Source: CAD feature listing. Evaluate the final solid. Frame: model axes, mm. Face numbers are marked on the shaded views. A direction names the side the tool comes from. Give positions to 0.01 mm unless a question says otherwise; leave off trailing zeros. Write each loop counter-clockwise with the first axis right and the second up, starting at its lowest first coordinate (ties: lowest second). Pieces come first, ordered by that corner, then holes. Notation, with made-up numbers: (-35, -6.75) -> (-14, -6.75) arc R16 cw to (-14, -2.75) -> close; hole circle Ø9 at (83, 49). An arc over 180 degrees is marked (long way). Use one line per item in the form item = value. Start each with the question number.
(1) Cut plane D-D, the plane y = 7.5. Output: boundary loops of the cut face in (x, z), and give its area (4 significant figures).
(2) Set-up query: the marked faces 4, 5 and 6. Return all of +Z, -Z, +X, -X, +Y, -Y with unobstructed straight access to the full face (end or side cutting, diameter ignored); none if empty.
(3) Cut plane B-B, the plane z = -4.25. Output: boundary loops of the cut face in (x, y).
(4) Cut plane A-A, the plane y = 0. Output: boundary loops of the cut face in (x, z), and give its area (3 significant figures).
(5) Cut plane C-C, the plane x = -4.5. Output: boundary loops of the cut face in (y, z), and give its area (3 significant figures).
(6) First-contact query: P1, Ø8, axis at x = -1.5, y = -5.5, coming from the -Z side; P2, Ø4, axis at x = -7.5, y = -6.5, coming from the -Z side; P3, Ø10, axis at x = -6.5, y = 7, coming from the -Z side; P4, Ø10, axis at x = 1, z = -8.5, coming from the -Y side. Flat tips, straight axial feed; report the tip coordinate or a pass-through.
(7) Draft query along Y for the marked faces 1, 2 and 3. Return one class per face: pulls with the +Y half, pulls with the -Y half, needs draft (parallel to the pull), parting line crosses it, or undercut.
(8) Material intervals for line 1 along Y through (x, z) = (0, 0.5); line 2 along X through (y, z) = (-3, -19.5); line 3 along X through (y, z) = (-7.5, 0.95), sorted ascending. Write a range as from..to.
from build123d import *

# Parameters (mm, degrees)
SKETCH1_W               = 16
SKETCH1_H               = 18
SKETCH1_W_2             = 12
SKETCH1_H_2             = 14
EXTRUDE_THIN1_DEPTH     = 2
BOSS_EXTRUDE3_DEPTH     = 2.2
CUT_EXTRUDE4_REACH      = 34.067
SKETCH10_W              = 0.2
SKETCH10_H              = 27.531461486
SKETCH5_R               = 3
CUT_EXTRUDE1_DEPTH      = 2
CUT_EXTRUDE1_DRAFT      = -35
MIRROR3_COPY_1_SKETCH_R = 3
MIRROR3_COPY_1_DEPTH    = 2
MIRROR3_COPY_1_DRAFT    = -35
SKETCH14_W              = 12
SKETCH14_H              = 4
BOSS_EXTRUDE5_DEPTH     = 14
CUT_EXTRUDE6_REACH      = 28.292
SKETCH15_R              = 6
CUT_EXTRUDE8_REACH      = 28.292
SKETCH19_R              = 0.5


with BuildPart() as part:
    # Sketch1 → Extrude-Thin1 (new, symmetric)
    with BuildSketch(Plane.XY):
        Rectangle(SKETCH1_W, SKETCH1_H)
        Rectangle(SKETCH1_W_2, SKETCH1_H_2, mode=Mode.SUBTRACT)
    extrude_thin1 = extrude(amount=EXTRUDE_THIN1_DEPTH, both=True)

    # Sketch4 → Boss-Extrude3 (add)
    with BuildSketch(Plane(origin=(8, 0, 0), x_dir=(0, 0, -1), z_dir=(1, 0, 0))):
        with BuildLine():
            Line((-2, 9), (15.5, 9))
            ThreePointArc((15.5, 9), (24.5, 0), (15.5, -9))
            Line((15.5, -9), (-2, -9))
            Line((-2, -9), (-2, 9))
        make_face()
    boss_extrude3 = extrude(amount=BOSS_EXTRUDE3_DEPTH)

    # Sketch10 → Cut-Extrude4 (cut, up to next)
    with BuildSketch(Plane(origin=(0, 9, 0), x_dir=(1, 0, 0), z_dir=(0, 1, 0)), mode=Mode.PRIVATE) as cut_extrude4_sk1:
        with Locations((8.1, 15.765730743)):
            Rectangle(SKETCH10_W, SKETCH10_H)
    cut_extrude4_tool1 = extrude(cut_extrude4_sk1.sketch, amount=-CUT_EXTRUDE4_REACH, mode=Mode.PRIVATE) & part.part
    cut_extrude4 = cut_extrude4_tool1.solids().sort_by_distance((8.1, 9, -15.765731))[0]
    add(cut_extrude4, mode=Mode.SUBTRACT)


with BuildPart() as cut_extrude1_tool:
    # Sketch5 → Cut-Extrude1 (with draft: the straight prism first)
    with BuildSketch(Plane.ZY.offset(-8.2)):
        with Locations((-15.5, 0)):
            Circle(SKETCH5_R)
    extrude(amount=-CUT_EXTRUDE1_DEPTH)
    # Cut-Extrude1: the draft: its side faces are tilted about the plane it starts from
    cut_extrude1_sides = [cut_extrude1_tool.faces().sort_by_distance(p)[0] for p in [
        (9.2, 0, -18.5),
    ]]
    draft(cut_extrude1_sides, Plane.ZY.offset(-8.2), CUT_EXTRUDE1_DRAFT)


with BuildPart() as part_1:
    add(part.part)

    # Cut-Extrude1: cut by cut_extrude1_tool
    add(cut_extrude1_tool.part, mode=Mode.SUBTRACT)

    # Mirror3: Extrude-Thin1, Boss-Extrude3, Cut-Extrude4 across plane
    add(extrude_thin1.mirror(Plane(origin=(0, 0, 0), x_dir=(0, 0, 1), z_dir=(1, 0, 0))))
    add(boss_extrude3.mirror(Plane(origin=(0, 0, 0), x_dir=(0, 0, 1), z_dir=(1, 0, 0))))
    add(cut_extrude4.mirror(Plane(origin=(0, 0, 0), x_dir=(0, 0, 1), z_dir=(1, 0, 0))), mode=Mode.SUBTRACT)


with BuildPart() as mirror3_copy_1_tool:
    # Mirror3 copy 1 sketch → Mirror3 copy 1 (with draft: the straight prism first)
    with BuildSketch(Plane(origin=(-8.2, 0, 0), x_dir=(0, 0, 1), z_dir=(1, 0, 0))):
        with Locations((-15.5, 0)):
            Circle(MIRROR3_COPY_1_SKETCH_R)
    extrude(amount=-MIRROR3_COPY_1_DEPTH)
    # Mirror3 copy 1: the draft: its side faces are tilted about the plane it starts from
    mirror3_copy_1_sides = [mirror3_copy_1_tool.faces().sort_by_distance(p)[0] for p in [
        (-9.2, 0, -18.5),
    ]]
    draft(mirror3_copy_1_sides, Plane(origin=(-8.2, 0, 0), x_dir=(0, 0, 1), z_dir=(1, 0, 0)), MIRROR3_COPY_1_DRAFT)


with BuildPart() as part_2:
    add(part_1.part)

    # Mirror3 copy 1: cut by mirror3_copy_1_tool
    add(mirror3_copy_1_tool.part, mode=Mode.SUBTRACT)

    # Sketch14 → Boss-Extrude5 (add)
    with BuildSketch(Plane(origin=(0, -7, 0), x_dir=(1, 0, 0), z_dir=(0, 1, 0))):
        Rectangle(SKETCH14_W, SKETCH14_H)
    extrude(amount=BOSS_EXTRUDE5_DEPTH)

    # Sketch15 → Cut-Extrude6 (cut, up to next)
    with BuildSketch(Plane(origin=(0, 0, -2), x_dir=(-1, 0, 0), z_dir=(0, 0, -1)), mode=Mode.PRIVATE) as cut_extrude6_sk1:
        Circle(SKETCH15_R)
    cut_extrude6_tool1 = extrude(cut_extrude6_sk1.sketch, amount=-CUT_EXTRUDE6_REACH, mode=Mode.PRIVATE) & part_2.part
    add(cut_extrude6_tool1.solids().sort_by_distance((0, 0, -2))[0], mode=Mode.SUBTRACT)

    # Sketch19 → Cut-Extrude8 (cut, up to next)
    with BuildSketch(Plane(origin=(0, 0, -2), x_dir=(-1, 0, 0), z_dir=(0, 0, -1)), mode=Mode.PRIVATE) as cut_extrude8_sk1:
        with Locations((0, 7.5)):
            Circle(SKETCH19_R)
    cut_extrude8_tool1 = extrude(cut_extrude8_sk1.sketch, amount=-CUT_EXTRUDE8_REACH, mode=Mode.PRIVATE) & part_2.part
    cut_extrude8 = cut_extrude8_tool1.solids().sort_by_distance((0, 7.5, -2))[0]
    add(cut_extrude8, mode=Mode.SUBTRACT)

    # Mirror8: Cut-Extrude8 across plane
    add(cut_extrude8.mirror(Plane.ZX), mode=Mode.SUBTRACT)

    # Mirror8 at the second plane: Cut-Extrude8 across plane
    add(cut_extrude8.mirror(Plane(origin=(0, 0, 0), x_dir=(0, 0, 1), z_dir=(1, 0, 0))), mode=Mode.SUBTRACT)


solid = part_2.part
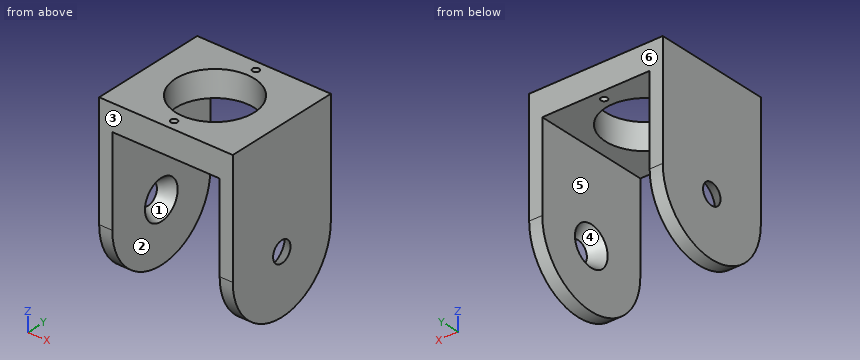
Geometry says:
q1.outline = (-10.2, -20.47) -> (-8.2, -20.47) -> (-8.2, -2) -> (-0.5, -2) -> (-0.5, 2) -> (-10.2, 2) -> close; (0.5, -2) -> (8.2, -2) -> (8.2, -20.47) -> (10.2, -20.47) -> (10.2, 2) -> (0.5, 2) -> close
q1.area = 151.5 mm^2
q2.face_4 = none
q2.face_5 = -Z, +Y, -Y
q2.face_6 = +Z, -Z, +X, -X, +Y
q3.outline = (-10.2, -9) -> (-8.2, -9) -> (-8.2, 9) -> (-10.2, 9) -> close; (8.2, -9) -> (10.2, -9) -> (10.2, 9) -> (8.2, 9) -> close
q4.outline = (-10.2, -24.5) -> (-8.2, -24.5) -> (-8.2, -18.5) -> (-10.2, -17.1) -> close; (-10.2, -13.9) -> (-8.2, -12.5) -> (-8.2, -2) -> (-6, -2) -> (-6, 2) -> (-10.2, 2) -> close; (6, -2) -> (8.2, -2) -> (8.2, -12.5) -> (10.2, -13.9) -> (10.2, 2) -> (6, 2) -> close; (8.2, -24.5) -> (10.2, -24.5) -> (10.2, -17.1) -> (8.2, -18.5) -> close
q4.area = 105 mm^2
q5.outline = (-9, -2) -> (-3.97, -2) -> (-3.97, 2) -> (-9, 2) -> close; (3.97, -2) -> (9, -2) -> (9, 2) -> (3.97, 2) -> close
q5.area = 40.3 mm^2
q6.P1 = -2
q6.P2 = -23.22
q6.P3 = -24.2
q6.P4 = through
q7.face_1 = undercut
q7.face_2 = needs draft
q7.face_3 = pulls with the -Y half
q8.line_1 = -9..-8, -7..-6, 6..7, 8..9
q8.line_2 = -10.2..-8.2, 8.2..10.2
q8.line_3 = -10.2..-0.5, 0.5..10.2
